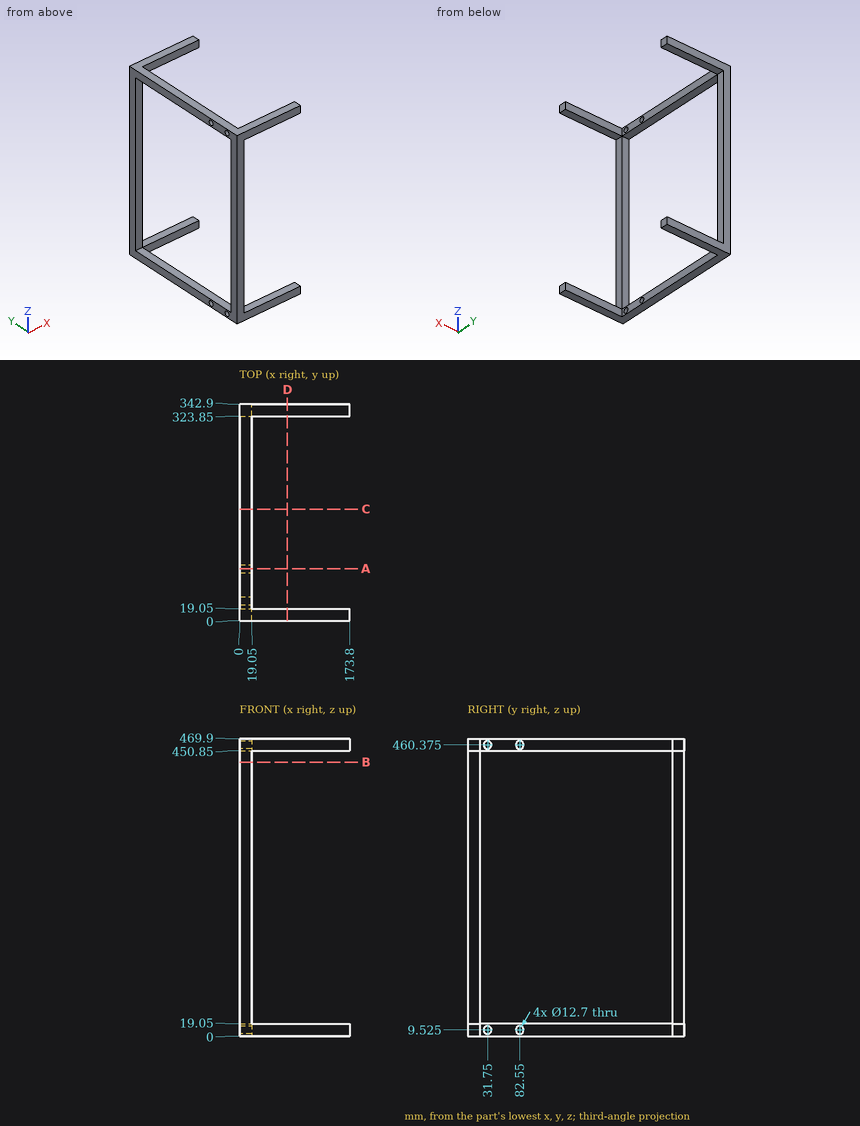
Print and shaded views of the part. All mm, measured from the part's lowest x, y and z. Round coordinates to 2 decimals unless told otherwise and drop trailing zeros. Write each loop counter-clockwise with the first axis right and the second up, starting at its lowest first coordinate (ties: lowest second). Pieces come first, ordered by that corner, then holes.
Item 1: Drop flat-ended pins along their axis: pin 1 Ø10 at (y, z) = (82.55, 9.525) entering from +X; pin 2 Ø5.5 at (y, z) = (233.5, 7.5) entering from +X. Give the stop position or say it passes through.
Results:
pin 1: passes through
pin 2: stops at x = 19.05
Item 2: Cut at D-D, the plane x = 75.5. Give the cut face in (y, z), plus the area to 3 significant figures.
Results:
outline: (0, 0) - (19.05, 0) - (19.05, 19.05) - (0, 19.05) - close; (0, 450.85) - (19.05, 450.85) - (19.05, 469.9) - (0, 469.9) - close; (323.85, 0) - (342.9, 0) - (342.9, 19.05) - (323.85, 19.05) - close; (323.85, 450.85) - (342.9, 450.85) - (342.9, 469.9) - (323.85, 469.9) - close
area: 1,450 mm2
Item 3: Cut at B-B, the plane z = 433. Give the cut face in (x, y).
Results:
outline: (0, 0) - (19.05, 0) - (19.05, 19.05) - (0, 19.05) - close; (0, 323.85) - (19.05, 323.85) - (19.05, 342.9) - (0, 342.9) - close
Item 4: Probe L1, parallel to Z at x = 9, y = 82; L2, parallel to Z at x = 6, y = 31; L3, parallel to Y at x = 9, z = 382.5. List the from-to ranges inside material, lowest first.
Results:
L1: z = 0 to 3.2, 15.85 to 19.05, 450.85 to 454.05, 466.7 to 469.9
L2: z = 0 to 3.22, 15.83 to 19.05, 450.85 to 454.07, 466.68 to 469.9
L3: y = 0 to 19.05, 323.85 to 342.9
Item 5: Cut at A-A, the plane y = 82.55. Count the separate pieces of the cut face and the enclosed holes in it, plus the area to 3 significant figures.
Results:
separate pieces: 4
enclosed holes: 0
area: 242 mm2
Item 6: Cut at C-C, the plane y = 176.5. Give the cut face in (x, z), plus the area to 3 significant figures.
Results:
outline: (0, 0) - (19.05, 0) - (19.05, 19.05) - (0, 19.05) - close; (0, 450.85) - (19.05, 450.85) - (19.05, 469.9) - (0, 469.9) - close
area: 726 mm2
